Read the model definition and answer for the solid it produces. Units are mm, in the model's axes. A direction names the side the tool comes from. Coordinates: 2 decimals unless noted, no trailing zeros. Order: outer loops, then holes, each group sorted by start corner. A loop starts at its lowest first (then second) coordinate and runs counter-clockwise, first axis right, second up. Notation, with made-up numbers: (33.25, 50.5) - (67.25, 50.5) arc R20 ccw to (67.25, 63.5) - close; hole circle Ø9 at (41, -22). An arc over 180 degrees is marked (long way). Answer as a JSON object with one key per item and string values. Group by question number.
from build123d import *

# Parameters (mm, degrees)
CROQUIS1_W                   = 55
CROQUIS1_H                   = 13
SALIENTE_EXTRUIR1_DEPTH      = 5
CROQUIS2_R                   = 2.5
CORTAR_EXTRUIR1_DEPTH        = 5
CROQUIS3_W                   = 26
CROQUIS3_H                   = 5
CORTAR_EXTRUIR2_DEPTH        = 5
SALIENTE_EXTRUIR2_DEPTH      = 5
SALIENTE_EXTRUIR2_DEPTH_BACK = 8
CROQUIS4_R                   = 14.25
CROQUIS5_R                   = 12
CORTAR_EXTRUIR3_DEPTH        = 1
CORTAR_EXTRUIR4_START        = -1
CROQUIS6_R                   = 12
CORTAR_EXTRUIR4_DEPTH        = 1
SALIENTE_EXTRUIR3_DEPTH      = 1
SALIENTE_EXTRUIR3_DEPTH_BACK = 12
SALIENTE_EXTRUIR4_DEPTH      = 13
CROQUIS9_R                   = 11
CORTAR_EXTRUIR5_DEPTH        = 13
CROQUIS10_W                  = 30.554627906
CROQUIS10_H                  = 17.725009208
CORTAR_EXTRUIR6_DEPTH        = 1.5
CROQUIS11_W                  = 31.627471091
CROQUIS11_H                  = 18.560833894
CORTAR_EXTRUIR7_DEPTH        = 1.5
CORTAR_EXTRUIR8_START        = -1.5
CROQUIS13_R                  = 12
CORTAR_EXTRUIR8_DEPTH        = 1.5
CROQUIS14_R                  = 12
CORTAR_EXTRUIR10_DEPTH       = 1.5
CORTAR_EXTRUIR11_START       = 5
CROQUIS15_R                  = 12
CORTAR_EXTRUIR11_DEPTH       = 5
CROQUIS16_R                  = 12
CORTAR_EXTRUIR12_DEPTH       = 5
CORTAR_EXTRUIR13_DEPTH       = 20
CORTAR_EXTRUIR14_DEPTH       = 36
CORTAR_EXTRUIR15_DEPTH       = 36
CORTAR_EXTRUIR16_DEPTH       = 23
CROQUIS22_R                  = 12
SALIENTE_EXTRUIR6_DEPTH      = 1.5
CROQUIS23_R                  = 14.25
SALIENTE_EXTRUIR7_DEPTH      = 1.5
SALIENTE_EXTRUIR9_DEPTH      = 5
SALIENTE_EXTRUIR10_DEPTH     = 5
SALIENTE_EXTRUIR11_START     = -1.5
SALIENTE_EXTRUIR11_DEPTH     = 1.5
SALIENTE_EXTRUIR12_START     = -1.5
SALIENTE_EXTRUIR12_DEPTH     = 1.5
SALIENTE_EXTRUIR13_START     = -10
CROQUIS30_R                  = 11.125
CROQUIS30_R_2                = 11
SALIENTE_EXTRUIR13_DEPTH     = 10
CROQUIS31_R                  = 11.125
CORTAR_EXTRUIR17_DEPTH       = 7
CROQUIS32_R                  = 11.25
CORTAR_EXTRUIR18_DEPTH       = 7


with BuildPart() as part:
    # Croquis1 → Saliente-Extruir1 (new body)
    with BuildSketch(Plane(origin=(0, 0, 0), x_dir=(1, 0, 0), z_dir=(0, 1, 0))):
        Rectangle(CROQUIS1_W, CROQUIS1_H)
    extrude(amount=SALIENTE_EXTRUIR1_DEPTH)

    # Croquis2 → Cortar-Extruir1 (cut)
    with BuildSketch(Plane(origin=(0, 5, 0), x_dir=(1, 0, 0), z_dir=(0, 1, 0))):
        with Locations(Location((-20.65, 0, 0), (0, 0, 270))):
            Circle(CROQUIS2_R)
        with Locations(Location((20.95, 0, 0), (0, 0, 270))):
            Circle(CROQUIS2_R)
    extrude(amount=-CORTAR_EXTRUIR1_DEPTH, mode=Mode.SUBTRACT)

    # Croquis3 → Cortar-Extruir2 (cut)
    with BuildSketch(Plane(origin=(0, 5, 0), x_dir=(1, 0, 0), z_dir=(0, 1, 0))):
        with Locations((0, 4)):
            Rectangle(CROQUIS3_W, CROQUIS3_H)
        with Locations((0, -4)):
            Rectangle(CROQUIS3_W, CROQUIS3_H)
    extrude(amount=-CORTAR_EXTRUIR2_DEPTH, mode=Mode.SUBTRACT)

    # Croquis4 → Saliente-Extruir2 (add, two sides: drawn at the far end of the back side and taken through both)
    with BuildSketch(Plane.XY.offset(1.5).offset(-SALIENTE_EXTRUIR2_DEPTH_BACK)):
        with Locations((0, 14.25)):
            Circle(CROQUIS4_R)
    extrude(amount=SALIENTE_EXTRUIR2_DEPTH + SALIENTE_EXTRUIR2_DEPTH_BACK)

    # Croquis5 → Cortar-Extruir3 (cut)
    with BuildSketch(Plane(origin=(0, 0, -6.5), x_dir=(-1, 0, 0), z_dir=(0, 0, -1))):
        with Locations((0, 14.25)):
            Circle(CROQUIS5_R)
    extrude(amount=-CORTAR_EXTRUIR3_DEPTH, mode=Mode.SUBTRACT)

    # Croquis6 → Cortar-Extruir4 (cut)
    with BuildSketch(Plane.XY.offset(6.5).offset(CORTAR_EXTRUIR4_START)):
        with Locations(Location((0, 14.25, 0), (0, 0, 180))):
            Circle(CROQUIS6_R)
    extrude(amount=CORTAR_EXTRUIR4_DEPTH, mode=Mode.SUBTRACT)

    # Croquis7 → Saliente-Extruir3 (add, two sides: drawn at the far end of the back side and taken through both)
    with BuildSketch(Plane.XY.offset(5.5).offset(-SALIENTE_EXTRUIR3_DEPTH_BACK)):
        Polygon((-12, 14.25), (-13, 0), (-14.25, 5), (-14.25, 14.25), align=None)
        Polygon((12, 14.25), (13, 0), (14.25, 5), (14.25, 14.25), align=None)
    extrude(amount=SALIENTE_EXTRUIR3_DEPTH + SALIENTE_EXTRUIR3_DEPTH_BACK)

    # Croquis8 → Saliente-Extruir4 (add)
    with BuildSketch(Plane.XY.offset(6.5)):
        Polygon((-10.839741694, 5), (-13.183687754, 5), (-12.649122807, 8.463153797), align=None)
        Polygon((12.728523578, 8.463153797), (12.649122807, 5), (10.839741694, 5), align=None)
    extrude(amount=-SALIENTE_EXTRUIR4_DEPTH)

    # Croquis9 → Cortar-Extruir5 (cut)
    with BuildSketch(Plane.XY.offset(5.5)):
        with Locations((0, 14.25)):
            Circle(CROQUIS9_R)
    extrude(amount=-CORTAR_EXTRUIR5_DEPTH, mode=Mode.SUBTRACT)

    # Croquis10 → Cortar-Extruir6 (cut)
    with BuildSketch(Plane(origin=(0, 0, -6.5), x_dir=(-1, 0, 0), z_dir=(0, 0, -1))):
        with Locations((1.027313953, 23.112504604)):
            Rectangle(CROQUIS10_W, CROQUIS10_H)
    extrude(amount=-CORTAR_EXTRUIR6_DEPTH, mode=Mode.SUBTRACT)

    # Croquis11 → Cortar-Extruir7 (cut)
    with BuildSketch(Plane.XY.offset(6.5)):
        with Locations((-1.563735546, 23.530416947)):
            Rectangle(CROQUIS11_W, CROQUIS11_H)
    extrude(amount=-CORTAR_EXTRUIR7_DEPTH, mode=Mode.SUBTRACT)

    # Croquis13 → Cortar-Extruir8 (cut)
    with BuildSketch(Plane.XY.offset(5).offset(CORTAR_EXTRUIR8_START)):
        with Locations((0, 14.25)):
            Circle(CROQUIS13_R)
    extrude(amount=CORTAR_EXTRUIR8_DEPTH, mode=Mode.SUBTRACT)

    # Croquis14 → Cortar-Extruir10 (cut)
    with BuildSketch(Plane(origin=(0, 0, -5), x_dir=(-1, 0, 0), z_dir=(0, 0, -1))):
        with Locations(Location((0, 14.25, 0), (0, 0, 180))):
            Circle(CROQUIS14_R)
    extrude(amount=-CORTAR_EXTRUIR10_DEPTH, mode=Mode.SUBTRACT)

    # Croquis15 → Cortar-Extruir11 (cut)
    with BuildSketch(Plane(origin=(0, 0, -3.5), x_dir=(-1, 0, 0), z_dir=(0, 0, -1)).offset(CORTAR_EXTRUIR11_START)):
        with Locations((0, 14.25)):
            Circle(CROQUIS15_R)
    extrude(amount=-CORTAR_EXTRUIR11_DEPTH, mode=Mode.SUBTRACT)

    # Croquis16 → Cortar-Extruir12 (cut)
    with BuildSketch(Plane.XY.offset(3.5)):
        with Locations(Location((0, 14.25, 0), (0, 0, 180))):
            Circle(CROQUIS16_R)
    extrude(amount=CORTAR_EXTRUIR12_DEPTH, mode=Mode.SUBTRACT)

    # Croquis17 → Cortar-Extruir13 (cut)
    with BuildSketch(Plane.XY.offset(5)):
        Polygon((-12, 14.25), (-13, 0), (13, 0), (12, 14.25), align=None)
    extrude(amount=CORTAR_EXTRUIR13_DEPTH, mode=Mode.SUBTRACT)

    # Croquis18 → Cortar-Extruir14 (cut)
    with BuildSketch(Plane.ZY.offset(14.25)):
        Polygon((5, 14.25), (6.5, 5), (6.5, 14.25), align=None)
    extrude(amount=-CORTAR_EXTRUIR14_DEPTH, mode=Mode.SUBTRACT)

    # Croquis19 → Cortar-Extruir15 (cut)
    with BuildSketch(Plane(origin=(14.25, 0, 0), x_dir=(0, 0, -1), z_dir=(1, 0, 0))):
        Polygon((5, 14.25), (6.5, 5), (6.5, 14.25), align=None)
    extrude(amount=-CORTAR_EXTRUIR15_DEPTH, mode=Mode.SUBTRACT)

    # Croquis20 → Cortar-Extruir16 (cut)
    with BuildSketch(Plane(origin=(0, 0, -5), x_dir=(-1, 0, 0), z_dir=(0, 0, -1))):
        Polygon((-12, 14.25), (-13, 0), (13, 0), (12, 14.25), align=None)
    extrude(amount=CORTAR_EXTRUIR16_DEPTH, mode=Mode.SUBTRACT)

    # Croquis22 → Saliente-Extruir6 (add)
    with BuildSketch(Plane.XY.offset(3.5)):
        with Locations(Location((0, 14.25, 0), (0, 0, 180))):
            Circle(CROQUIS22_R)
    extrude(amount=SALIENTE_EXTRUIR6_DEPTH)

    # Croquis23 → Saliente-Extruir7 (add)
    with BuildSketch(Plane.XY.offset(5)):
        with Locations((0, 14.25)):
            Circle(CROQUIS23_R)
    extrude(amount=SALIENTE_EXTRUIR7_DEPTH)

    # Croquis24 → Saliente-Extruir9 (add)
    with BuildSketch(Plane.XY.offset(1.5)):
        with BuildLine():
            Line((-10.839741694, 5), (-12.649122807, 5))
            Line((-12.649122807, 5), (-13, 0))
            Line((-13, 0), (0, 0))
            ThreePointArc((0, 0), (-5.968668193, 1.310235705), (-10.839741694, 5))
        make_face()
    extrude(amount=SALIENTE_EXTRUIR9_DEPTH)

    # Croquis26 → Saliente-Extruir10 (add)
    with BuildSketch(Plane.XY.offset(1.5)):
        with BuildLine():
            Line((0, 0), (13, 0))
            Line((13, 0), (12.649122807, 5))
            Line((12.649122807, 5), (10.839741694, 5))
            ThreePointArc((10.839741694, 5), (5.968668193, 1.310235705), (0, 0))
        make_face()
    extrude(amount=SALIENTE_EXTRUIR10_DEPTH)

    # Croquis27 → Saliente-Extruir11 (add)
    with BuildSketch(Plane.XY.offset(6.5).offset(SALIENTE_EXTRUIR11_START)):
        with BuildLine():
            Line((-12.649122807, 5), (-10.839741694, 5))
            ThreePointArc((-10.839741694, 5), (-13.370280834, 9.320690674), (-14.25, 14.25))
            Line((-14.25, 14.25), (-14.25, 5))
            Line((-14.25, 5), (-12.649122807, 5))
        make_face()
    extrude(amount=SALIENTE_EXTRUIR11_DEPTH)

    # Croquis28 → Saliente-Extruir12 (add)
    with BuildSketch(Plane.XY.offset(6.5).offset(SALIENTE_EXTRUIR12_START)):
        with BuildLine():
            ThreePointArc((14.25, 14.25), (13.370280834, 9.320690674), (10.839741694, 5))
            Line((10.839741694, 5), (12.649122807, 5))
            Line((12.649122807, 5), (14.25, 5))
            Line((14.25, 5), (14.25, 14.25))
        make_face()
    extrude(amount=SALIENTE_EXTRUIR12_DEPTH)

    # Croquis30 → Saliente-Extruir13 (add)
    with BuildSketch(Plane(origin=(0, 0, -3.5), x_dir=(-1, 0, 0), z_dir=(0, 0, -1)).offset(SALIENTE_EXTRUIR13_START)):
        with Locations((0, 14.25)):
            Circle(CROQUIS30_R)
        with Locations(Location((0, 14.25, 0), (0, 0, 180))):
            Circle(CROQUIS30_R_2, mode=Mode.SUBTRACT)
    extrude(amount=SALIENTE_EXTRUIR13_DEPTH)

    # Croquis31 → Cortar-Extruir17 (cut)
    with BuildSketch(Plane(origin=(0, 0, -3.5), x_dir=(-1, 0, 0), z_dir=(0, 0, -1))):
        with Locations((0, 14.25)):
            Circle(CROQUIS31_R)
    extrude(amount=-CORTAR_EXTRUIR17_DEPTH, mode=Mode.SUBTRACT)

    # Croquis32 → Cortar-Extruir18 (cut)
    with BuildSketch(Plane(origin=(0, 0, -3.5), x_dir=(-1, 0, 0), z_dir=(0, 0, -1))):
        with Locations((0, 14.25)):
            Circle(CROQUIS32_R)
    extrude(amount=-CORTAR_EXTRUIR18_DEPTH, mode=Mode.SUBTRACT)


solid = part.part
1. A cutting plane is placed at D-D on y = 12.5. Write down the section's boundary in (x, z), and give its area (3 significant figures).
2. A cutting plane is placed at C-C on z = 5.25. Write down the section's boundary in (x, y).
3. Straight lines are drawn through the part: L1, parallel to X at y = 1, z = 0; L2, parallel to X at y = 4.5, z = -3.75; L3, parallel to Z at x = 5.5, y = 15.5. For each, find the intervals that lie inside material, in ascending order.
4. For a pull along Y with two mould halves and no side action, classify faces 5 (the flat face through (13.39, 9.69, -5.74)), 6 (the cylindrical face through (5.537, 24.896, -4.26)), 7 (the flat face through (20, 3, -6.5)), 8 (the flat face through (0, 14, 3.5)) as pulls with the +Y half, pulls with the -Y half, needs draft (parallel to the pull), parting line crosses it, or undercut.
5. Given pin 1 (2 mm diameter, centred on y = 17, z = -4, fed in from -X); pin 2 (3 mm diameter, centred on x = 14.5, y = 15.5, fed in from +Z); pin 3 (8 mm diameter, centred on x = -11.5, y = 13.5, fed in from -Z); pin 4 (7.5 mm diameter, centred on y = 11, z = 1, fed in from -X), each flat-ended and moving along its own axis, determine where each tip first touches the part or whether it passes through.
6. A cutting plane is placed at B-B on z = -0.5. Write down the section's boundary in (x, y).
7. A cutting plane is placed at A-A on x = 20.95. Write down the section's boundary in (y, z).
8. For faces 1 (the flat face through (-21, 5, -3)), 2 (the flat face through (-12, 5, -3)), 3 (the flat face through (-2, 27, -5)), 4 (the flat face through (14.25, 10, 0)), determine the directions among +Z, -Z, +X, -X, +Y, -Y from which every point of the face is accessible in a straight line to the end or side of a thin tool.
Derived:
{
 "1": {"outline": "(-14.25, -5.28) - (-12.12, -5.28) - (-12.12, -5) - (-11.87, -5) - (-11.87, -3.5) - (-11.11, -3.5) - (-11.11, 3.5) - (11.11, 3.5) - (11.11, -3.5) - (11.87, -3.5) - (11.87, -5) - (12.12, -5) - (12.12, -5.28) - (14.25, -5.28) - (14.25, 6.5) - (-14.25, 6.5) - close", "area": "138 mm2"},
 "2": {"outline": "(-27.5, 0) - (27.5, 0) - (27.5, 5) - (14.25, 5) - (14.25, 14.25) arc R14.25 ccw to (-14.25, 14.25) - (-14.25, 5) - (-27.5, 5) - close"},
 "3": {"L1": "x = -27.5 to -23.15, -18.15 to 18.45, 23.45 to 27.5", "L2": "x = -27.5 to -12.68, -10.39 to -7, 7 to 10.39, 12.68 to 27.5", "L3": "z = 3.5 to 6.5"},
 "4": {"face 5": "pulls with the +Y half", "face 6": "undercut", "face 7": "needs draft", "face 8": "undercut"},
 "5": {"pin 1": "stops at x = -14.14", "pin 2": "stops at z = 6.5", "pin 3": "stops at z = -5.76", "pin 4": "stops at x = -14.25"},
 "6": {"outline": "(-27.5, 0) - (-23.1, 0) - (-23.1, 5) - (-27.5, 5) - close; (-18.2, 0) - (18.5, 0) - (18.5, 5) - (14.25, 5) - (14.25, 14.25) arc R14.25 ccw to (-14.25, 14.25) - (-14.25, 5) - (-18.2, 5) - close; (23.4, 0) - (27.5, 0) - (27.5, 5) - (23.4, 5) - close; hole circle Ø22.5 at (0, 14.25)"},
 "7": {"outline": "(0, -6.5) - (5, -6.5) - (5, -2.5) - (0, -2.5) - close; (0, 2.5) - (5, 2.5) - (5, 6.5) - (0, 6.5) - close"},
 "8": {"face 1": "+Z, -Z, -X, +Y", "face 2": "-Z, -Y", "face 3": "-Z, +X, -X, +Y", "face 4": "+Z, -Z, +X, +Y"}
}
